Source: CAD feature listing. Evaluate the final solid. Frame: model axes, mm. A direction names the side the tool comes from. Round coordinates to 2 decimals unless told otherwise and drop trailing zeros. Loops run counter-clockwise (first coordinate to the right, second up) from the corner with the lowest first, then second, coordinate; pieces in that order, holes last. Notation, with made-up numbers: M -3,30 L 51,30 A8 ccw 51,43 Z; hole C -30,82.25 d6. An arc over 180 degrees is marked long. Write each question's results on one line, items separated by ' | '. Start each with the question number.
1. Ray query, line 1 (X direction, y = 3, z = -22.86); line 2 (Z direction, x = 50, y = 6.25); line 3 (Z direction, x = 69.85, y = 4). Return the intervals inside material, ascending.
2. Section A-A on x = 69.85. Output: boundary loops of the cut face in (y, z), and give its area (3 significant figures).
3. Set-up query: faces 4 (the flat face through (41, 3, 3.615)), 5 (the cylindrical face through (19.22, 3.13, 11.16)), 6 (the cylindrical face through (10.37, 3.13, 12.32)). Return all of +Z, -Z, +X, -X, +Y, -Y with unobstructed straight access to the full face (end or side cutting, diameter ignored); none if empty.
4. Draft query along Z for faces 1 (the flat face through (49, 3, 6.439)), 2 (the flat face through (16.51, 3, -20)), 3 (the cylindrical face through (63.06, 3.22, -0.08)). Return one class per face: released by +Z, released by -Z, zero draft, split by the parting line, or undercut.
5. Contact query for flat-ended pins moving along their axis: pin 1 Ø3 at (y, z) = (2, 2) entering from -X; pin 2 Ø10 at (x, z) = (49, 16) entering from +Y; pin 3 Ø3 at (x, y) = (25, 3.5) entering from -Z; pin 4 Ø1.9 at (x, y) = (50, 4.5) entering from +Z. Output: stop coordinate, or through.
6. Section B-B on z = -22.86. Output: boundary loops of the cut face in (x, y), and give its area (3 significant figures).
7. Section C-C on y = 2.5. Give the number of separate pieces and of enclosed holes in the cut face, and give its area (3 significant figures).
from build123d import *

# Parameters (mm, degrees)
SKETCH1_R                = 22.225
SKETCH1_R_2              = 15.875
BOSS_EXTRUDE1_DEPTH      = 6.35
BOSS_EXTRUDE2_DEPTH      = 6.35
F_0_257_DIAMETER_HOLE1_D = 6.5278
SKETCH6_W                = 65.552410467
SKETCH6_H                = 82.171101747
CUT_EXTRUDE2_DEPTH       = 7.35
FILLET2_R                = 2.54
SKETCH9_R                = 2.15265
BOSS_EXTRUDE3_DEPTH      = 6.35
FILLET4_R                = 1.27
CUT_EXTRUDE3_DEPTH       = 7.35


with BuildPart() as part:
    # Sketch1 → Boss-Extrude1 (new body)
    with BuildSketch(Plane(origin=(0, 0, 0), x_dir=(1, 0, 0), z_dir=(0, 1, 0))):
        Circle(SKETCH1_R)
        Circle(SKETCH1_R_2, mode=Mode.SUBTRACT)
    extrude(amount=BOSS_EXTRUDE1_DEPTH)

    # Sketch2 → Boss-Extrude2 (add)
    with BuildSketch(Plane(origin=(0, 6.35, 0), x_dir=(1, 0, 0), z_dir=(0, 1, 0))):
        with BuildLine():
            Line((75.953359527, -6.4389), (38.518839527, -6.4389))
            Line((38.518839527, -6.4389), (17.590769706, -6.4389))
            Line((17.590769706, -6.4389), (17.590769706, 6.4389))
            Line((17.590769706, 6.4389), (38.518839527, 6.4389))
            Line((38.518839527, 6.4389), (75.953359527, 6.4389))
            ThreePointArc((75.953359527, 6.4389), (80.443487588, 4.579028061), (82.303359527, 0.0889))
            Line((82.303359527, 0.0889), (82.303359527, -0.0889))
            ThreePointArc((82.303359527, -0.0889), (80.443487588, -4.579028061), (75.953359527, -6.4389))
        make_face()
    extrude(amount=-BOSS_EXTRUDE2_DEPTH)

    # F (0.257) Diameter Hole1 (through all)
    with Locations(Plane(origin=(0, 6.35, 0), x_dir=(1, 0, 0), z_dir=(0, 1, 0))):
        with Locations((69.85, 0)):
            Hole(F_0_257_DIAMETER_HOLE1_D / 2)

    # Sketch6 → Cut-Extrude2 (cut, through all)
    with BuildSketch(Plane(origin=(0, 6.35, 0), x_dir=(1, 0, 0), z_dir=(0, 1, 0))):
        with Locations((-22.616205234, -1.153387837)):
            Rectangle(SKETCH6_W, SKETCH6_H)
    extrude(amount=-CUT_EXTRUDE2_DEPTH, mode=Mode.SUBTRACT)

    # Fillet2
    fillet2_edges = [part.edges().sort_by_distance(p)[0] for p in [
        (10.16, 3.175, -12.197951672),
        (10.16, 3.175, 12.197951672),
    ]]
    fillet(fillet2_edges, radius=FILLET2_R)

    # Sketch9 → Boss-Extrude3 (add)
    with BuildSketch(Plane(origin=(0, 6.35, 0), x_dir=(1, 0, 0), z_dir=(0, 1, 0))):
        Polygon((10.16, 19.766765669), (10.16, 26.116765669), (16.51, 26.116765669), (16.51, 14.878525633), align=None)
        with Locations((13.335, 22.86)):
            Circle(SKETCH9_R, mode=Mode.SUBTRACT)
    boss_extrude3 = extrude(amount=-BOSS_EXTRUDE3_DEPTH)

    # Mirror1: Boss-Extrude3 across plane
    add(boss_extrude3.mirror(Plane.XY))

    # Fillet4
    fillet4_edges = [part.edges().sort_by_distance(p)[0] for p in [
        (21.271840348, 3.175, 6.4389),
        (21.271840348, 3.175, -6.4389),
        (16.51, 3.175, 14.878525633),
        (16.51, 3.175, 26.116765669),
        (10.16, 3.175, 26.116765669),
        (16.51, 3.175, -14.878525633),
        (10.16, 3.175, -26.116765669),
        (16.51, 3.175, -26.116765669),
    ]]
    fillet(fillet4_edges, radius=FILLET4_R)

    # Sketch11 → Cut-Extrude3 (cut, through all)
    with BuildSketch(Plane(origin=(0, 6.35, 0), x_dir=(1, 0, 0), z_dir=(0, 1, 0))):
        with BuildLine():
            Line((59.445816997, -3.615471241), (22.916160789, -3.615471241))
            ThreePointArc((22.916160789, -3.615471241), (19.300689548, 0), (22.916160789, 3.615471241))
            Line((22.916160789, 3.615471241), (59.445816997, 3.615471241))
            ThreePointArc((59.445816997, 3.615471241), (63.061288238, 0), (59.445816997, -3.615471241))
        make_face()
    extrude(amount=-CUT_EXTRUDE3_DEPTH, mode=Mode.SUBTRACT)


solid = part.part
Taken from the geometry:
1) line 1: 10.16 to 11.18, 15.49 to 16.51 | line 2: -6.44 to -3.62, 3.62 to 6.44 | line 3: -6.44 to -3.26, 3.26 to 6.44
2) outline: M 0,-6.44 L 6.35,-6.44 L 6.35,-3.26 L 0,-3.26 Z; M 0,3.26 L 6.35,3.26 L 6.35,6.44 L 0,6.44 Z | area: 40.3 mm^2
3) face 4: +Y, -Y | face 5: +Z, +X, +Y, -Y | face 6: -X, +Y, -Y
4) face 1: released by +Z | face 2: zero draft | face 3: undercut
5) pin 1: x = 15.48 | pin 2: through | pin 3: z = -6.44 | pin 4: z = 6.44
6) outline: M 10.16,0 L 11.18,0 L 11.18,6.35 L 10.16,6.35 Z; M 15.49,0 L 16.51,0 L 16.51,6.35 L 15.49,6.35 Z | area: 13.0 mm^2
7) separate pieces: 1 | enclosed holes: 4 | area: 743 mm^2
